Input: part model. Units: mm. Frame: model coordinates. A direction names the side the tool comes from. Coordinates: 2 decimals unless noted, no trailing zeros. Write each loop counter-clockwise with the first axis right and the second up, starting at its lowest first coordinate (ties: lowest second). Pieces come first, ordered by that corner, then holes.
from build123d import *

# Parameters (mm, degrees)
ESQUISSE1_W             = 52
ESQUISSE1_H             = 202
BOSS_EXTRU_1_DEPTH      = 102
COQUE1_T                = -1
ESQUISSE2_W             = 50
ESQUISSE2_H             = 200
BOSS_EXTRU_2_DEPTH      = 1
ESQUISSE3_R             = 4.5
ENL_V_MAT_EXTRU_1_DEPTH = 1


with BuildPart() as part:
    # Esquisse1 → Boss.-Extru.1 (new body)
    with BuildSketch(Plane.XY):
        Rectangle(ESQUISSE1_W, ESQUISSE1_H)
    extrude(amount=BOSS_EXTRU_1_DEPTH)

    # Coque1
    coque1_openings = [part.faces().sort_by_distance(p)[0] for p in [
        (0, 0, 102),
    ]]
    offset(amount=COQUE1_T, openings=coque1_openings, kind=Kind.INTERSECTION)

    # Esquisse2 → Boss.-Extru.2 (add)
    with BuildSketch(Plane.XY.offset(102)):
        Rectangle(ESQUISSE2_W, ESQUISSE2_H)
    extrude(amount=-BOSS_EXTRU_2_DEPTH)

    # Esquisse3 → Enlèv. mat.-Extru.1 (cut)
    with BuildSketch(Plane.XY.offset(102)):
        with Locations((0, -81)):
            Circle(ESQUISSE3_R)
        with Locations((0, -51)):
            Circle(ESQUISSE3_R)
    extrude(amount=-ENL_V_MAT_EXTRU_1_DEPTH, mode=Mode.SUBTRACT)


solid = part.part
Item 1: Section query D-D, the plane y = -51. Return loops of the section in (x, z).
Item 2: Access query for faces 1 (the face through (26, -1, 50)), 2 (the face through (25, -1, 50)), 3 (the face through (-0.59, -76.54, 101.51)). Directions: +Z, -Z, +X, -X, +Y, -Y. A direction counts if a zero-diameter tool reaches every point of the face in a straight line with its end or side. Return the directions, or none.
Item 3: Section query C-C, the plane y = 83.5. Return loops of the section in (x, z), then the cut area to 3 significant figures.
Item 4: Pull-direction query (X, two-part tool) for faces 4 (the face through (-26, -1, 50)), 5 (the face through (0, 1, 101)), 6 (the face through (0, 101, 50)); classes: released by +X, released by -X, zero draft, split by the parting line, or undercut.
Item 5: Section query A-A, the plane x = 0. Return loops of the section in (y, z), then the cut area to 3 significant figures.
Item 6: Section query B-B, the plane z = 88. Return loops of the section in (x, y), then the cut area to 3 significant figures.
Item 7: Material intervals for line 1 (Y direction, x = 0, z = 101.55); line 2 (Z direction, x = 1, y = 35.5); line 3 (Y direction, x = 12.5, z = 55.5), sorted ascending.
Item 8: Pin query (flat end, axial travel): pin 1 Ø14.5 at (x, y) = (0, -51) entering from -Z; pin 2 Ø8 at (x, y) = (0, -81) entering from +Z. Return the tip coordinate at first contact, or that it passes through.
The answers:
1. outline: (-26, 0) - (26, 0) - (26, 102) - (4.5, 102) - (4.5, 101) - (25, 101) - (25, 1) - (-25, 1) - (-25, 101) - (-4.5, 101) - (-4.5, 102) - (-26, 102) - close
2. face 1: +Z, -Z, +X, +Y, -Y
2. face 2: none
2. face 3: +Z
3. outline: (-26, 0) - (26, 0) - (26, 102) - (-26, 102) - close; hole (-25, 1) - (25, 1) - (25, 101) - (-25, 101) - close
3. area: 304 mm2
4. face 4: released by -X
4. face 5: undercut
4. face 6: zero draft
5. outline: (-101, 0) - (101, 0) - (101, 102) - (-46.5, 102) - (-46.5, 101) - (100, 101) - (100, 1) - (-100, 1) - (-100, 101) - (-85.5, 101) - (-85.5, 102) - (-101, 102) - close; (-76.5, 101) - (-55.5, 101) - (-55.5, 102) - (-76.5, 102) - close
5. area: 586 mm2
6. outline: (-26, -101) - (26, -101) - (26, 101) - (-26, 101) - close; hole (-25, -100) - (25, -100) - (25, 100) - (-25, 100) - close
6. area: 504 mm2
7. line 1: y = -101 to -85.5, -76.5 to -55.5, -46.5 to 101
7. line 2: z = 0 to 1, 101 to 102
7. line 3: y = -101 to -100, 100 to 101
8. pin 1: stops at z = 0
8. pin 2: stops at z = 1
